from build123d import *

# Parameters (mm, degrees)
BASE_FLANGE2_DEPTH      = 25.4
CUT_EXTRUDE1_DEPTH      = 61.989758362
CUT_EXTRUDE1_DEPTH_BACK = 61.989758362
SKETCH10_R              = 3.175


# Sheet-metal steps are written as plain solids
with BuildPart() as part:
    # Sketch1 → Base-Flange2 (new body)
    with BuildSketch(Plane.XY):
        with BuildLine():
            Line((-22.225, -50.8), (-22.225, -3.937))
            ThreePointArc((-22.225, -3.937), (-21.071879398, -1.153120602), (-18.288, 0))
            Line((-18.288, 0), (18.288, 0))
            ThreePointArc((18.288, 0), (21.071879398, -1.153120602), (22.225, -3.937))
            Line((22.225, -3.937), (22.225, -50.8))
            Line((22.225, -50.8), (19.05, -50.8))
            Line((19.05, -50.8), (19.05, -3.937))
            ThreePointArc((19.05, -3.937), (18.826815367, -3.398184633), (18.288, -3.175))
            Line((18.288, -3.175), (-18.288, -3.175))
            ThreePointArc((-18.288, -3.175), (-18.826815367, -3.398184633), (-19.05, -3.937))
            Line((-19.05, -3.937), (-19.05, -50.8))
            Line((-19.05, -50.8), (-22.225, -50.8))
        make_face()
    extrude(amount=BASE_FLANGE2_DEPTH)

    # Sketch10 → Cut-Extrude1 (cut, two sides: drawn at the far end of the back side and taken through both)
    with BuildSketch(Plane(origin=(0, 0, 0), x_dir=(0, 0, -1), z_dir=(1, 0, 0)).offset(-CUT_EXTRUDE1_DEPTH_BACK)):
        with Locations(Location((-17.4625, -27.3685, 0), (0, 0, 180))):
            Circle(SKETCH10_R)
    extrude(amount=CUT_EXTRUDE1_DEPTH + CUT_EXTRUDE1_DEPTH_BACK, mode=Mode.SUBTRACT)


solid = part.part
Design review of the part built by this model. Coordinates are the model's own, in mm. A direction names the side the tool comes from. Give positions to 0.01 mm unless a question says otherwise; leave off trailing zeros. Write each loop counter-clockwise with the first axis right and the second up, starting at its lowest first coordinate (ties: lowest second). Pieces come first, ordered by that corner, then holes. Notation, with made-up numbers: M 1.5,-31.75 L 33.5,-31.75 A34 cw 33.5,5.25 Z; hole C -7,-7 d7. An arc over 180 degrees is marked long. Answer as a JSON object with one key per item and string values. Group by question number.
1) We need section B-B (z = 16.5). Give the boundary of the cut face in (x, y) (3 decimals).
2) Tool access review of faces 1 (the face through (0, 0, 13)), 2 (the face through (-19.05, -27, 13)): name each direction out of +Z, -Z, +X, -X, +Y, -Y from which nothing blocks a thin tool from reaching the whole face with its end or side.
3) We need section D-D (z = 2.75). Give the boundary of the cut face in (x, y) (3 decimals).
4) Mouldability with a two-part tool opening along X and no side actions: class faces 3 (the face through (-21, -50.8, 13)), 4 (the face through (19.05, -28, 13)), 5 (the face through (21.04, -1.12, 12.52)) as released by +X, released by -X, zero draft, split by the parting line, or undercut.
5) Clearance check with flat-ended pins moving along their axes: pin 1 Ø10 at (x, z) = (-5, 4) entering from -Y (3 decimals); pin 2 Ø4 at (y, z) = (-27.37, 17.46) entering from -X; pin 3 Ø7.5 at (y, z) = (-27.37, 17.46) entering from +X (3 decimals). State where each tip first meets the part, or that it passes through.
6) We need section A-A (y = -44). Give the boundary of the cut face in (x, z) (3 decimals), and give its area (3 significant figures).
7) For line 1 along X through (y, z) = (-26, 22) (3 decimals); line 2 along Y through (x, z) = (-6.5, 18.75) (3 decimals), list the stretches that pass through material, from the lowest coordinate up.
8) We need section C-C (y = -25.5). Give the boundary of the cut face in (x, z) (3 decimals), and give its area (3 significant figures).
Answer key:
{
 "1": {"outline": "M -22.225,-50.8 L -19.05,-50.8 L -19.05,-30.394 L -22.225,-30.394 Z; M -22.225,-24.343 L -19.05,-24.343 L -19.05,-3.937 A0.762 cw -18.288,-3.175 L 18.288,-3.175 A0.762 cw 19.05,-3.937 L 19.05,-24.343 L 22.225,-24.343 L 22.225,-3.937 A3.937 ccw 18.288,0 L -18.288,0 A3.937 ccw -22.225,-3.937 Z; M 19.05,-50.8 L 22.225,-50.8 L 22.225,-30.394 L 19.05,-30.394 Z"},
 "2": {"face 1": "+Z, -Z, +X, -X, +Y", "face 2": "+Z, -Z, -Y"},
 "3": {"outline": "M -22.225,-50.8 L -19.05,-50.8 L -19.05,-3.937 A0.762 cw -18.288,-3.175 L 18.288,-3.175 A0.762 cw 19.05,-3.937 L 19.05,-50.8 L 22.225,-50.8 L 22.225,-3.937 A3.937 ccw 18.288,0 L -18.288,0 A3.937 ccw -22.225,-3.937 Z"},
 "4": {"face 3": "zero draft", "face 4": "undercut", "face 5": "released by +X"},
 "5": {"pin 1": "stops at y = -3.175", "pin 2": "passes through", "pin 3": "stops at x = 22.225"},
 "6": {"outline": "M -22.225,0 L -19.05,0 L -19.05,25.4 L -22.225,25.4 Z; M 19.05,0 L 22.225,0 L 22.225,25.4 L 19.05,25.4 Z", "area": "161 mm²"},
 "7": {"line 1": "x = -22.225 to -19.05, 19.05 to 22.225", "line 2": "y = -3.175 to 0"},
 "8": {"outline": "M -22.225,0 L -19.05,0 L -19.05,14.896 L -22.225,14.896 Z; M -22.225,20.029 L -19.05,20.029 L -19.05,25.4 L -22.225,25.4 Z; M 19.05,0 L 22.225,0 L 22.225,14.896 L 19.05,14.896 Z; M 19.05,20.029 L 22.225,20.029 L 22.225,25.4 L 19.05,25.4 Z", "area": "129 mm²"}
}
